from build123d import *

# Parameters (mm, degrees)
F0_W     = 8.45
F0_H     = 8
F1_DEPTH = 4
F2_W     = 18.45
F2_H     = 18
F3_DEPTH = 2
F4_R     = 5
F5_DEPTH = 10
F6_R     = 2.9
F7_DEPTH = 16.001
F8_R     = 2
F9_R     = 0.5


with BuildPart() as f1:
    # F0 (on Top) → F1 (new body)
    with BuildSketch(Plane.XY):
        Rectangle(F0_W, F0_H)
    extrude(amount=F1_DEPTH)

    # F2 (on face) → F3 (join)
    with BuildSketch(Plane.XY.offset(4)):
        Rectangle(F2_W, F2_H)
    extrude(amount=F3_DEPTH)

    # F4 (on face) → F5 (join)
    with BuildSketch(Plane.XY.offset(6)):
        Circle(F4_R)
    extrude(amount=F5_DEPTH)

    # F6 (on face) → F7 (cut, through all)
    with BuildSketch(Plane.XY.offset(16)):
        Circle(F6_R)
    extrude(amount=-F7_DEPTH, mode=Mode.SUBTRACT)

    # F8
    f8_edges = [f1.edges().sort_by_distance(p)[0] for p in [
        (-9.225, 9, 5),
        (9.225, 9, 5),
        (9.225, -9, 5),
        (-9.225, -9, 5),
        (-5, 0, 16),
    ]]
    fillet(f8_edges, radius=F8_R)

    # F9
    f9_edges = [f1.edges().sort_by_distance(p)[0] for p in [
        (-2.9, 0, 16),
        (-2.9, 0, 0),
        (-4.225, 0, 0),
        (0, 4, 0),
        (0, -4, 0),
        (4.225, 0, 0),
    ]]
    fillet(f9_edges, radius=F9_R)


solid = f1.part
Could you check a few things on this model? Use its own coordinates, in mm. A direction names the side the tool comes from. Give positions to 0.01 mm unless a question says otherwise; leave off trailing zeros. Order: outer loops, then holes, each group sorted by start corner. A loop starts at its lowest first (then second) coordinate and runs counter-clockwise, first axis right, second up.
1. We'd pull the mould along Y, two halves only. Please class faces 1 (the flat face through (0, 4, 2)), 2 (the flat face through (0, -9, 5)), 3 (the cylindrical face through (1.559, 2.445, 8.077)): pulls with the +Y half, pulls with the -Y half, needs draft (parallel to the pull), parting line crosses it, or undercut.
2. Suppose I cut it at C-C (x = -5.5). List the corners of the cut face in (y, z) for me, plus the area to 3 significant figures.
3. Suppose I cut it at A-A (z = 3). List the corners of the cut face in (x, y) for me (3 decimals), plus the area to 3 significant figures.
4. Suppose I cut it at D-D (z = 13). List the corners of the cut face in (x, y) for me, plus the area to 3 significant figures.
5. Suppose I cut it at B-B (y = 6.5). List the corners of the cut face in (x, z) for me (3 decimals).
6. Will these pins go through, and if not, where does the flat tip stop? P1, Ø3, axis at x = -1.5, z = 2, coming from the +Y side; P2, Ø1.5, axis at x = -5, z = 7, coming from the -Y side; P3, Ø1.8, axis at x = 0, z = 3, coming from the -Y side.
7. I need wall thicknesses on L1, parallel to X at y = 0, z = 5.5 (3 decimals); L2, parallel to Y at x = 0, z = 8.75; L3, parallel to Z at x = 5, y = 6. Which ranges of each line are inside material? Lowest first, please.
8. For faces 4 (the cylindrical face through (-8.655, -8.399, 5.014)), 5 (the flat face through (4.225, 0, 2)), 6 (the flat face through (-4, -4, 6)), 7 (the flat face through (-4.225, 0, 2)), 8 (the flat face through (0, -4, 2)), which set-ups out of +Z, -Z, +X, -X, +Y, -Y let a thin tool reach every point of the face, with its end or its side?
Solved:
1. face 1: pulls with the +Y half
1. face 2: pulls with the -Y half
1. face 3: undercut
2. outline: (-9, 4) - (9, 4) - (9, 6) - (-9, 6) - close
2. area: 36.0 mm2
3. outline: (-4.225, -4) - (4.225, -4) - (4.225, 4) - (-4.225, 4) - close; hole circle Ø5.8 at (0, 0)
3. area: 41.2 mm2
4. outline: circle Ø10 at (0, 0); hole circle Ø5.8 at (0, 0)
4. area: 52.1 mm2
5. outline: (-9.225, 4) - (9.225, 4) - (9.225, 6) - (-9.225, 6) - close
6. P1: stops at y = 4
6. P2: stops at y = -2.63
6. P3: stops at y = -4
7. L1: x = -9.225 to -2.9, 2.9 to 9.225
7. L2: y = -5 to -2.9, 2.9 to 5
7. L3: z = 4 to 6
8. face 4: +Z, -Z, -X, -Y
8. face 5: -Z, +X, +Y, -Y
8. face 6: +Z
8. face 7: -Z, -X, +Y, -Y
8. face 8: -Z, +X, -X, -Y
